```python
from build123d import *

# Parameters (mm, degrees)
ESBO_O1_R                = 3.1
ESBO_O1_R_2              = 1.55
RESSALTO_EXTRUS_O1_DEPTH = 16.74
BOSS_EXTRUDE1_DEPTH      = 16.74
SKETCH2_W                = 6.2
SKETCH2_H                = 1.935
BOSS_EXTRUDE2_DEPTH      = 7.715
BOSS_EXTRUDE3_DEPTH      = 6.2
SKETCH5_W                = 16.74
SKETCH5_H                = 5.66650546
BOSS_EXTRUDE4_DEPTH      = 2
SKETCH6_W                = 16.74
SKETCH6_H                = 4.529470895
BOSS_EXTRUDE5_DEPTH      = 1
FILLET1_R                = 1
FILLET4_R                = 1
M3_CLEARANCE_HOLE1_D     = 3.2


with BuildPart() as part:
    # Esboço1 → Ressalto-extrusão1 (new body)
    with BuildSketch(Plane.XY):
        with Locations((16.016666667, 16.016666667)):
            Circle(ESBO_O1_R)
        with Locations((16.016666667, 16.016666667)):
            Circle(ESBO_O1_R_2, mode=Mode.SUBTRACT)
    extrude(amount=RESSALTO_EXTRUS_O1_DEPTH)

    # Sketch1 → Boss-Extrude1 (add)
    with BuildSketch(Plane(origin=(0, 0, 0), x_dir=(-1, 0, 0), z_dir=(0, 0, -1))):
        with BuildLine():
            Line((-12.916666667, 16.016666667), (-12.916666667, 19.634677588))
            Line((-12.916666667, 19.634677588), (-19.116666667, 19.634677588))
            Line((-19.116666667, 19.634677588), (-19.116666667, 16.016666667))
            ThreePointArc((-19.116666667, 16.016666667), (-16.016666667, 19.116666667), (-12.916666667, 16.016666667))
        make_face()
    extrude(amount=-BOSS_EXTRUDE1_DEPTH)

    # Sketch2 → Boss-Extrude2 (add)
    with BuildSketch(Plane(origin=(0, 19.634677588, 0), x_dir=(1, 0, 0), z_dir=(0, 1, 0))):
        with Locations((16.016666667, -0.9675)):
            Rectangle(SKETCH2_W, SKETCH2_H)
        with Locations((16.016666667, -15.7725)):
            Rectangle(SKETCH2_W, SKETCH2_H)
    extrude(amount=BOSS_EXTRUDE2_DEPTH)

    # Sketch4 → Boss-Extrude3 (add)
    with BuildSketch(Plane.ZY.offset(-12.916666667)):
        Polygon((1.935, 27.349677588), (1.935, 25.349677588), (2.619300497, 25.349677588), align=None)
        Polygon((14.120699503, 25.349677588), (14.805, 27.349677588), (14.805, 25.349677588), align=None)
    extrude(amount=-BOSS_EXTRUDE3_DEPTH)

    # Sketch5 → Boss-Extrude4 (add)
    with BuildSketch(Plane(origin=(19.116666667, 0, 0), x_dir=(0, 0, -1), z_dir=(1, 0, 0))):
        with Locations((-8.37, 18.849919397)):
            Rectangle(SKETCH5_W, SKETCH5_H)
    extrude(amount=BOSS_EXTRUDE4_DEPTH)

    # Sketch6 → Boss-Extrude5 (add)
    with BuildSketch(Plane.ZY.offset(-12.916666667)):
        with Locations((8.37, 18.281402115)):
            Rectangle(SKETCH6_W, SKETCH6_H)
    extrude(amount=BOSS_EXTRUDE5_DEPTH)

    # Fillet1
    fillet1_edges = [part.edges().sort_by_distance(p)[0] for p in [
        (21.116666667, 21.683172127, 8.37),
        (21.116666667, 18.849919397, 0),
        (21.116666667, 16.016666667, 8.37),
        (21.116666667, 18.849919397, 16.74),
        (16.016666667, 27.349677588, 0),
        (16.016666667, 27.349677588, 1.935),
        (16.016666667, 27.349677588, 16.74),
        (16.016666667, 27.349677588, 14.805),
        (19.116666667, 21.683172127, 15.7725),
        (12.916666667, 20.546137562, 15.7725),
        (12.916666667, 20.546137562, 0.9675),
        (19.116666667, 21.683172127, 0.9675),
        (12.916666667, 16.016666667, 8.37),
        (19.116666667, 16.016666667, 8.37),
    ]]
    fillet(fillet1_edges, radius=FILLET1_R - 0.0001)  # a hair under: the kernel refuses the full size

    # Fillet4
    fillet4_edges = [part.edges().sort_by_distance(p)[0] for p in [
        (11.916666667, 16.016666667, 8.37),
    ]]
    fillet(fillet4_edges, radius=FILLET4_R)

    # M3 Clearance Hole1 (through all)
    with Locations(Plane(origin=(0, 0, 0), x_dir=(-1, 0, 0), z_dir=(0, 0, -1))):
        with Locations((-16.016666667, 16.016666667)):
            Hole(M3_CLEARANCE_HOLE1_D / 2)


solid = part.part
```
Source: CAD feature listing. Evaluate the final solid. Frame: model axes, mm. A direction names the side the tool comes from. Give positions to 0.01 mm unless a question says otherwise; leave off trailing zeros. Loops run counter-clockwise (first coordinate to the right, second up) from the corner with the lowest first, then second, coordinate; pieces in that order, holes last. Notation, with made-up numbers: (-33.5, 49.25) -> (-1.5, 49.25) arc R26 ccw to (-1.5, 87.25) -> close; hole circle Ø5 at (42.5, 85.25). An arc over 180 degrees is marked (long way). Use a Markdown table: item, result. Add a question column.
(1) Section query A-A (y = 20.25). Output: boundary loops of the cut face in (x, z) (3 decimals), then the cut area to 3 significant figures.
(2) Section query C-C (y = 14.75). Output: boundary loops of the cut face in (x, z), then the cut area to 3 significant figures.
(3) Pull-direction query (X, two-part tool) for faces 5 (the face through (16, 20, 16.74)), 6 (the face through (19.117, 21, 8)), 7 (the face through (19.37, 15.8, 8.49)); classes: +X half, -X half, draft (parallel to the pull), parting line (faces both ways), or undercut.
(4) Section query B-B (x = 15.5). Output: boundary loops of the cut face in (y, z) (3 decimals).
(5) Ray query, line 1 (Z direction, x = 16.25, y = 20.5) (3 decimals); line 2 (Y direction, x = 16, z = 1); line 3 (Y direction, x = 17, z = 11). Return the intervals inside material, ascending.
(6) First-contact query: pin 1 Ø0.8 at (y, z) = (24.5, 1) entering from -X; pin 2 Ø0.8 at (y, z) = (25.5, 15.5) entering from +X; pin 3 Ø0.5 at (x, z) = (12, 5) entering from +Y; pin 4 Ø1.9 at (x, y) = (16.02, 16.02) entering from -Z (3 decimals). Flat tips, straight axial feed; report the tip coordinate or a pass-through.
(7) Section query D-D (x = 13.5). Output: boundary loops of the cut face in (y, z) (3 decimals), then the cut area to 3 significant figures.
(8) Access query for faces 1 (the face through (16.06, 27.158, 14.931)), 2 (the face through (19.117, 25, 1)), 3 (the face through (21.117, 19, 8)), 4 (the face through (12.917, 24, 1)). Directions: +Z, -Z, +X, -X, +Y, -Y. A direction counts if a zero-diameter tool reaches every point of the face in a straight line with its end or side. Return the directions, or none.
Checked values:
| question | item | result |
|---|---|---|
| 1 | outline | (11.917, 0) -> (20.117, 0) arc R1 ccw to (21.117, 1) -> (21.117, 15.74) arc R1 ccw to (20.117, 16.74) -> (11.917, 16.74) -> close; hole (12.917, 1.935) -> (19.117, 1.935) -> (19.117, 14.805) -> (12.917, 14.805) -> close |
| 1 | area | 73.8 mm^2 |
| 2 | outline | (13.19, 0) -> (15.04, 0) -> (15.04, 16.74) -> (13.19, 16.74) -> close; (16.99, 0) -> (18.85, 0) -> (18.85, 16.74) -> (16.99, 16.74) -> close |
| 2 | area | 62.0 mm^2 |
| 3 | face 5 | draft |
| 3 | face 6 | undercut |
| 3 | face 7 | +X half |
| 4 | outline | (12.96, 0) -> (14.502, 0) -> (14.502, 16.74) -> (12.96, 16.74) -> close; (17.531, 0) -> (26.35, 0) arc R1 ccw to (27.35, 1) -> (27.35, 1.22) arc R1 ccw to (26.673, 2.166) -> (25.35, 2.619) -> (25.35, 1.935) -> (19.635, 1.935) -> (19.635, 14.805) -> (25.35, 14.805) -> (25.35, 14.121) -> (26.673, 14.574) arc R1 ccw to (27.35, 15.52) -> (27.35, 15.74) arc R1 ccw to (26.35, 16.74) -> (17.531, 16.74) -> close |
| 5 | line 1 | 0 to 1.935, 14.805 to 16.74 |
| 5 | line 2 | 12.92 to 14.42, 17.62 to 27.35 |
| 5 | line 3 | 13.08 to 14.75, 17.28 to 19.63 |
| 6 | pin 1 | x = 12.92 |
| 6 | pin 2 | x = 19.12 |
| 6 | pin 3 | y = 20.55 |
| 6 | pin 4 | through |
| 7 | outline | (14.207, 0) -> (26.35, 0) arc R1 ccw to (27.35, 1) -> (27.35, 1.22) arc R1 ccw to (26.673, 2.166) -> (25.35, 2.619) -> (25.35, 1.935) -> (19.635, 1.935) -> (19.635, 14.805) -> (25.35, 14.805) -> (25.35, 14.121) -> (26.673, 14.574) arc R1 ccw to (27.35, 15.52) -> (27.35, 15.74) arc R1 ccw to (26.35, 16.74) -> (14.207, 16.74) -> close |
| 7 | area | 121 mm^2 |
| 8 | face 1 | +X, -X, +Y |
| 8 | face 2 | +Z, -Z, +X, +Y |
| 8 | face 3 | +Z, -Z, +X, +Y, -Y |
| 8 | face 4 | +Z, -Z, -X, +Y |
